Could you check a few things on this model? Use its own coordinates, in mm. A direction names the side the tool comes from. Give positions to 0.01 mm unless a question says otherwise; leave off trailing zeros. Order: outer loops, then holes, each group sorted by start corner. A loop starts at its lowest first (then second) coordinate and runs counter-clockwise, first axis right, second up. Notation, with made-up numbers: M -36.5,1 L 22.5,1 A26 ccw 22.5,30 Z; hole C -26,19.25 d11. An arc over 180 degrees is marked long. Return JSON: item names as keys, results as strings. Group by question number.
```python
from build123d import *

# Parameters (mm, degrees)
SKETCH1_R           = 7
BOSS_EXTRUDE1_DEPTH = 3.175
SKETCH2_R           = 1.65
CUT_EXTRUDE1_DEPTH  = 10


with BuildPart() as part:
    # Sketch1 → Boss-Extrude1 (new body)
    with BuildSketch(Plane(origin=(0, 0, 0), x_dir=(1, 0, 0), z_dir=(0, 1, 0))):
        with BuildLine():
            Line((0, 0), (120, 0))
            ThreePointArc((120, 0), (136, 16), (120, 32))
            Line((120, 32), (0, 32))
            ThreePointArc((0, 32), (-16, 16), (0, 0))
        make_face()
        with Locations(Location((0, 16, 0), (0, 0, 270))):
            Circle(SKETCH1_R, mode=Mode.SUBTRACT)
        with Locations(Location((120, 16, 0), (0, 0, 270))):
            Circle(SKETCH1_R, mode=Mode.SUBTRACT)
        with BuildLine():
            Line((56.368317676, 16.477323769), (64.971964222, 28.764604433))
            ThreePointArc((64.971964222, 28.764604433), (67.061056942, 29.132967845), (67.429420354, 27.043875124))
            Line((67.429420354, 27.043875124), (58.825773809, 14.75659446))
            ThreePointArc((58.825773809, 14.75659446), (56.736681088, 14.388231048), (56.368317676, 16.477323769))
        make_face(mode=Mode.SUBTRACT)
    extrude(amount=BOSS_EXTRUDE1_DEPTH)

    # Sketch2 → Cut-Extrude1 (cut)
    with BuildSketch(Plane(origin=(0, 3.175, 0), x_dir=(1, 0, 0), z_dir=(0, 1, 0))):
        with Locations(Location((120, 27.313708499, 0), (0, 0, 270))):
            Circle(SKETCH2_R)
        with Locations(Location((108.686291501, 16, 0), (0, 0, 270))):
            Circle(SKETCH2_R)
        with Locations(Location((120, 4.686291501, 0), (0, 0, 270))):
            Circle(SKETCH2_R)
        with Locations(Location((131.313708499, 16, 0), (0, 0, 270))):
            Circle(SKETCH2_R)
        with Locations(Location((-11.313708499, 16, 0), (0, 0, 270))):
            Circle(SKETCH2_R)
        with Locations(Location((0, 27.313708499, 0), (0, 0, 270))):
            Circle(SKETCH2_R)
        with Locations(Location((11.313708499, 16, 0), (0, 0, 270))):
            Circle(SKETCH2_R)
        with Locations(Location((0, 4.686291501, 0), (0, 0, 270))):
            Circle(SKETCH2_R)
    extrude(amount=-CUT_EXTRUDE1_DEPTH, mode=Mode.SUBTRACT)


solid = part.part
```
1. If we mould it in two halves opening along X, with no side actions, what happens to faces 3 (the cylindrical face through (-11.946, 1.61, -14.476)), 4 (the cylindrical face through (-16, 2, -16)), 5 (the flat face through (61, 2, -32))? For each: pulls with the +X half, pulls with the -X half, needs draft (parallel to the pull), parting line crosses it, or undercut.
2. Imagine slicing it at C-C, the plane z = -20. Please give me the cut outline in (x, y) (3 decimals), plus the area to 3 significant figures.
3. For pin 1 (3 mm diameter, centred on x = -11.31, z = -16, fed in from -Y); pin 2 (1 mm diameter, centred on y = 1.5, z = -3.5, fed in from +X), each with a flat end and sliding along its axis, tell me the tip position at first contact or that it passes through.
4. Which directions (+Z, -Z, +X, -X, +Y, -Y) give clear straight access to the entire face, cutting with the end or side of a thin tool? Please do faces 1 (the flat face through (63.19, 1.57, -20.99)), 2 (the flat face through (59, 3.175, -13)).
5. Imagine slicing it at A-A, the plane x = -4. Please give me the cut outline in (y, z) (3 decimals).
6. I need wall thicknesses on L1, parallel to X at y = 1.15, z = -27; L2, parallel to X at y = 0.35, z = -22; L3, parallel to Z at x = 11.5, y = 2.55. Which ranges of each line are inside material? Lowest first, please. Write a range as from..to.
7. Imagine slicing it at B-B, the plane y = 0.65. Count the separate pieces of the cut face and the enclosed holes in it, plus the area to 3 significant figures.
Values:
{
 "1": {"face 3": "undercut", "face 4": "pulls with the -X half", "face 5": "needs draft"},
 "2": {"outline": "M -15.492,0 L -5.745,0 L -5.745,3.175 L -15.492,3.175 Z; M 5.745,0 L 58.835,0 L 58.835,3.175 L 5.745,3.175 Z; M 62.497,0 L 114.255,0 L 114.255,3.175 L 62.497,3.175 Z; M 125.745,0 L 135.492,0 L 135.492,3.175 L 125.745,3.175 Z", "area": "395 mm²"},
 "3": {"pin 1": "passes through", "pin 2": "stops at x = 130.58"},
 "4": {"face 1": "+Y, -Y", "face 2": "+Z, -Z, +X, -X, +Y"},
 "5": {"outline": "M 0,-31.492 L 3.175,-31.492 L 3.175,-21.745 L 0,-21.745 Z; M 0,-10.255 L 3.175,-10.255 L 3.175,-0.508 L 0,-0.508 Z"},
 "6": {"L1": "x = -11.62..-1.62, 1.62..63.74, 67.4..118.38, 121.62..131.62", "L2": "x = -14.83..-3.61, 3.61..60.24, 63.9..116.39, 123.61..134.83", "L3": "z = -32..-17.64, -14.36..0"},
 "7": {"separate pieces": "1", "enclosed holes": "11", "area": "4,220 mm²"}
}
